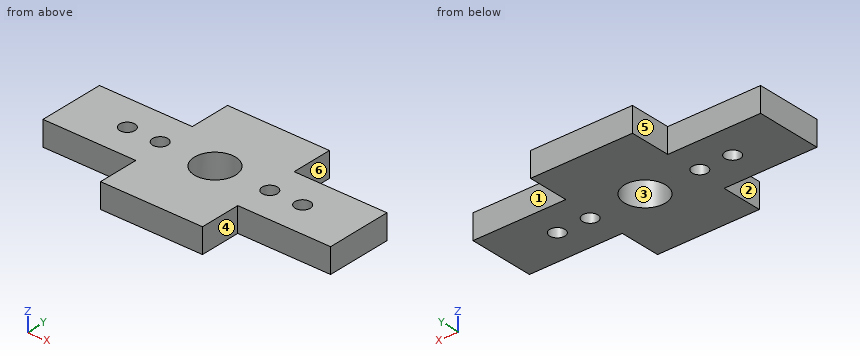
from build123d import *

# Parameters (mm, degrees)
ESQUISSE1_R        = 2.5
ESQUISSE1_R_2      = 0.925
BOSS_EXTRU_1_DEPTH = 3


with BuildPart() as part:
    # Esquisse1 → Boss.-Extru.1 (new body)
    with BuildSketch(Plane.XY):
        Polygon((-17.5, -4), (-17.5, 4), (-6.2, 4), (-6.2, 9), (6.2, 9), (6.2, 4), (17.5, 4), (17.5, -4), (6.2, -4), (6.2, -9), (-6.2, -9), (-6.2, -4), align=None)
        Circle(ESQUISSE1_R, mode=Mode.SUBTRACT)
        with Locations((6.67, 0)):
            Circle(ESQUISSE1_R_2, mode=Mode.SUBTRACT)
        with Locations((10.67, 0)):
            Circle(ESQUISSE1_R_2, mode=Mode.SUBTRACT)
        with Locations((-6.67, 0)):
            Circle(ESQUISSE1_R_2, mode=Mode.SUBTRACT)
        with Locations((-10.67, 0)):
            Circle(ESQUISSE1_R_2, mode=Mode.SUBTRACT)
    extrude(amount=BOSS_EXTRU_1_DEPTH)


solid = part.part
Can you work these out from the model? Positions are in its coordinate system, mm. Face numbers are marked on the shaded views. A direction names the side the tool comes from. Coordinates: 2 decimals unless noted, no trailing zeros. Write each loop counter-clockwise with the first axis right and the second up, starting at its lowest first coordinate (ties: lowest second). Pieces come first, ordered by that corner, then holes.
Q1. For P1, Ø1.5, axis at x = -10.5, z = 1, coming from the -Y side; P2, Ø1.5, axis at x = -6.67, y = 0, coming from the -Z side; P3, Ø0.9, axis at y = -7, z = 2, coming from the +X side; P4, Ø2.5, axis at x = -10.67, y = 0, coming from the -Z side, each with a flat end and sliding along its axis, tell me the tip position at first contact or that it passes through.
Results found:
P1: stops at y = -4
P2: passes through
P3: stops at x = 6.2
P4: stops at z = 0
Q2. Imagine slicing it at A-A, the plane x = 10.67. List the corners of the cut face in (y, z) for me (3 decimals), plus the area to 4 significant figures.
Results found:
outline: (-4, 0) - (-0.925, 0) - (-0.925, 3) - (-4, 3) - close; (0.925, 0) - (4, 0) - (4, 3) - (0.925, 3) - close
area: 18.45 mm2
Q3. Imagine slicing it at D-D, the plane y = -5.75. List the corners of the cut face in (x, z) for me, plus the area to 3 significant figures.
Results found:
outline: (-6.2, 0) - (6.2, 0) - (6.2, 3) - (-6.2, 3) - close
area: 37.2 mm2
Q4. Imagine slicing it at C-C, the plane x = -2. List the corners of the cut face in (y, z) for me.
Results found:
outline: (-9, 0) - (-1.5, 0) - (-1.5, 3) - (-9, 3) - close; (1.5, 0) - (9, 0) - (9, 3) - (1.5, 3) - close
Q5. If we mould it in two halves opening along X, with no side actions, what happens to the marked faces 1, 2 and 3? For each: +X half, -X half, draft (parallel to the pull), parting line (faces both ways), or undercut.
Results found:
face 1: draft
face 2: -X half
face 3: undercut
Q6. Please list where these lines run through material, in increasing order: L1, parallel to Y at x = -10.67, z = 1.25 (3 decimals); L2, parallel to Y at x = 0, z = 1.1; L3, parallel to Y at x = -13.5, z = 1.05.
Results found:
L1: y = -4 to -0.925, 0.925 to 4
L2: y = -9 to -2.5, 2.5 to 9
L3: y = -4 to 4
Q7. Imagine slicing it at B-B, the plane z = 0.9. List the corners of the cut face in (x, y) for me (3 decimals), plus the area to 3 significant figures.
Results found:
outline: (-17.5, -4) - (-6.2, -4) - (-6.2, -9) - (6.2, -9) - (6.2, -4) - (17.5, -4) - (17.5, 4) - (6.2, 4) - (6.2, 9) - (-6.2, 9) - (-6.2, 4) - (-17.5, 4) - close; hole circle Ø1.85 at (-10.67, 0); hole circle Ø1.85 at (-6.67, 0); hole circle Ø5 at (0, 0); hole circle Ø1.85 at (6.67, 0); hole circle Ø1.85 at (10.67, 0)
area: 374 mm2
Q8. Which directions (+Z, -Z, +X, -X, +Y, -Y) give clear straight access to the entire face, cutting with the end or side of a thin tool? Please do the marked faces 4, 5 and 6.
Results found:
face 4: +Z, -Z, +X, -Y
face 5: +Z, -Z, -X, +Y
face 6: +Z, -Z, +X, +Y
